```python
from build123d import *

# Parameters (mm, degrees)
SKETCH1_W               = 450
SKETCH1_H               = 280
BOSS_EXTRUDE1_DEPTH     = 95
FILLET1_R               = 10
FILLET2_R               = 5
CUT_EXTRUDE1_DEPTH      = 89
BOSS_EXTRUDE2_REACH     = 283.514
MIRROR2_COPY_1_REACH    = 283.514
FILLET4_R               = 1
SKETCH7_R               = 4
CUT_EXTRUDE2_DEPTH      = 40
MIRROR4_COPY_1_SKETCH_R = 4
MIRROR4_COPY_1_DEPTH    = 40
SKETCH8_R               = 2.25
SKETCH8_W               = 47
SKETCH8_H               = 26.9
CUT_EXTRUDE3_DEPTH      = 10
SKETCH10_R              = 2.53
SLOTS_FOR_LEDS_DEPTH    = 10
SKETCH11_R              = 12
SKETCH11_R_2            = 1.6
CUT_EXTRUDE4_DEPTH      = 10
SKETCH12_R              = 12
SKETCH12_R_2            = 1.6
CUT_EXTRUDE5_DEPTH      = 10


with BuildPart() as part:
    # Sketch1 → Boss-Extrude1 (new body)
    with BuildSketch(Plane(origin=(0, 0, 0), x_dir=(1, 0, 0), z_dir=(0, 1, 0))):
        Rectangle(SKETCH1_W, SKETCH1_H)
    extrude(amount=BOSS_EXTRUDE1_DEPTH)

    # Fillet1
    fillet1_edges = [part.edges().sort_by_distance(p)[0] for p in [
        (225, 47.5, 140),
        (-225, 47.5, 140),
        (-225, 47.5, -140),
        (225, 47.5, -140),
    ]]
    fillet(fillet1_edges, radius=FILLET1_R)

    # Fillet2
    fillet2_edges = [part.edges().sort_by_distance(p)[0] for p in [
        (-225, 0, 0),
        (225, 0, 0),
        (0, 0, 140),
        (0, 0, -140),
        (-222.071067812, 0, 137.071067812),
        (222.071067812, 0, 137.071067812),
        (222.071067812, 0, -137.071067812),
        (-222.071067812, 0, -137.071067812),
    ]]
    fillet(fillet2_edges, radius=FILLET2_R)

    # Sketch3 → Cut-Extrude1 (cut)
    with BuildSketch(Plane(origin=(0, 95, 0), x_dir=(1, 0, 0), z_dir=(0, 1, 0))):
        with BuildLine():
            Line((220, -130), (220, 130))
            ThreePointArc((220, 130), (218.535533906, 133.535533906), (215, 135))
            Line((215, 135), (-215, 135))
            ThreePointArc((-215, 135), (-218.535533906, 133.535533906), (-220, 130))
            Line((-220, 130), (-220, -130))
            ThreePointArc((-220, -130), (-218.535533906, -133.535533906), (-215, -135))
            Line((-215, -135), (215, -135))
            ThreePointArc((215, -135), (218.535533906, -133.535533906), (220, -130))
        make_face()
    extrude(amount=-CUT_EXTRUDE1_DEPTH, mode=Mode.SUBTRACT)

    # Sketch5 → Boss-Extrude2 (add, up to next)
    with BuildSketch(Plane(origin=(0, 95, 0), x_dir=(1, 0, 0), z_dir=(0, 1, 0)), mode=Mode.PRIVATE) as boss_extrude2_sk1:
        with BuildLine():
            Line((-205, 135), (-215, 135))
            ThreePointArc((-215, 135), (-218.535533906, 133.535533906), (-220, 130))
            Line((-220, 130), (-220, 120))
            ThreePointArc((-220, 120), (-209.393398282, 124.393398282), (-205, 135))
        make_face()
    boss_extrude2_tool1 = extrude(boss_extrude2_sk1.sketch, amount=-BOSS_EXTRUDE2_REACH, mode=Mode.PRIVATE) - part.part
    boss_extrude2 = boss_extrude2_tool1.solids().sort_by_distance((-213.469442, 95, -128.469442))[0]
    add(boss_extrude2)

    # Mirror1: Boss-Extrude2 across plane
    add(boss_extrude2.mirror(Plane.XY))

    # Mirror2: Boss-Extrude2 across plane
    add(boss_extrude2.mirror(Plane(origin=(0, 0, 0), x_dir=(0, 0, 1), z_dir=(1, 0, 0))))

    # Mirror2 copy 1 sketch → Mirror2 copy 1 (add, up to next)
    with BuildSketch(Plane(origin=(0, 95, 0), x_dir=(-1, 0, 0), z_dir=(0, 1, 0)), mode=Mode.PRIVATE) as mirror2_copy_1_sk1:
        with BuildLine():
            Line((-205, 135), (-215, 135))
            ThreePointArc((-215, 135), (-218.535533906, 133.535533906), (-220, 130))
            Line((-220, 130), (-220, 120))
            ThreePointArc((-220, 120), (-209.393398282, 124.393398282), (-205, 135))
        make_face()
    mirror2_copy_1_tool1 = extrude(mirror2_copy_1_sk1.sketch, amount=-MIRROR2_COPY_1_REACH, mode=Mode.PRIVATE) - part.part
    add(mirror2_copy_1_tool1.solids().sort_by_distance((213.469442, 95, 128.469442))[0])

    # Fillet4
    fillet4_edges = [part.edges().sort_by_distance(p)[0] for p in [
        (-220, 6, 0),
        (-209.393398282, 6, 124.393398282),
        (0, 6, 135),
        (209.393398282, 6, 124.393398282),
        (220, 6, 0),
        (209.393398282, 6, -124.393398282),
        (0, 6, -135),
        (-209.393398282, 6, -124.393398282),
    ]]
    fillet(fillet4_edges, radius=FILLET4_R)

    # Sketch7 → Cut-Extrude2 (cut)
    with BuildSketch(Plane(origin=(0, 95, 0), x_dir=(1, 0, 0), z_dir=(0, 1, 0))):
        with Locations(Location((-215, 130, 0), (0, 0, 270))):
            Circle(SKETCH7_R)
    cut_extrude2 = extrude(amount=-CUT_EXTRUDE2_DEPTH, mode=Mode.SUBTRACT)

    # Mirror3: Cut-Extrude2 across plane
    add(cut_extrude2.mirror(Plane.XY), mode=Mode.SUBTRACT)

    # Mirror4: Cut-Extrude2 across plane
    add(cut_extrude2.mirror(Plane(origin=(0, 0, 0), x_dir=(0, 0, 1), z_dir=(1, 0, 0))), mode=Mode.SUBTRACT)

    # Mirror4 copy 1 sketch → Mirror4 copy 1 (cut)
    with BuildSketch(Plane(origin=(0, 95, 0), x_dir=(-1, 0, 0), z_dir=(0, 1, 0))):
        with Locations(Location((-215, 130, 0), (0, 0, 270))):
            Circle(MIRROR4_COPY_1_SKETCH_R)
    extrude(amount=-MIRROR4_COPY_1_DEPTH, mode=Mode.SUBTRACT)

    # Sketch8 → Cut-Extrude3 (cut)
    with BuildSketch(Plane.XY.offset(140)):
        with Locations((-183, 35)):
            Circle(SKETCH8_R)
        with Locations((-127, 35)):
            Circle(SKETCH8_R)
        with Locations((-155, 35)):
            Rectangle(SKETCH8_W, SKETCH8_H)
    extrude(amount=-CUT_EXTRUDE3_DEPTH, mode=Mode.SUBTRACT)

    # Sketch10 → Slots for LEDs (cut)
    with BuildSketch(Plane(origin=(0, 0, -140), x_dir=(-1, 0, 0), z_dir=(0, 0, -1))):
        with Locations((-17, 75)):
            Circle(SKETCH10_R)
        with Locations((-2, 75)):
            Circle(SKETCH10_R)
        with Locations((13, 75)):
            Circle(SKETCH10_R)
        with Locations((28, 75)):
            Circle(SKETCH10_R)
        with Locations((43, 75)):
            Circle(SKETCH10_R)
        with Locations((58, 75)):
            Circle(SKETCH10_R)
    extrude(amount=-SLOTS_FOR_LEDS_DEPTH, mode=Mode.SUBTRACT)

    # Sketch11 → Cut-Extrude4 (cut)
    with BuildSketch(Plane.XY.offset(140)):
        with Locations((63.955734546, 69.39400536)):
            Circle(SKETCH11_R)
        with Locations((73.455734546, 41.39400536)):
            Circle(SKETCH11_R_2)
        with Locations((54.455734546, 17.39400536)):
            Circle(SKETCH11_R_2)
        with Locations((113.955734546, 69.39400536)):
            Circle(SKETCH11_R)
        with Locations((113.955734546, 29.39400536)):
            Circle(SKETCH11_R)
        with Locations((63.955734546, 29.39400536)):
            Circle(SKETCH11_R)
        with Locations((73.455734546, 81.39400536)):
            Circle(SKETCH11_R_2)
        with Locations((54.455734546, 57.39400536)):
            Circle(SKETCH11_R_2)
        with Locations((123.455734546, 41.39400536)):
            Circle(SKETCH11_R_2)
        with Locations((104.455734546, 17.39400536)):
            Circle(SKETCH11_R_2)
        with Locations((123.455734546, 81.39400536)):
            Circle(SKETCH11_R_2)
        with Locations((104.455734546, 57.39400536)):
            Circle(SKETCH11_R_2)
    extrude(amount=-CUT_EXTRUDE4_DEPTH, mode=Mode.SUBTRACT)

    # Sketch12 → Cut-Extrude5 (cut)
    with BuildSketch(Plane(origin=(0, 0, -140), x_dir=(-1, 0, 0), z_dir=(0, 0, -1))):
        with Locations((-67.078371633, 71.762757401)):
            Circle(SKETCH12_R)
        with Locations((-80.078371633, 84.762757401)):
            Circle(SKETCH12_R_2)
        with Locations((-54.078371633, 58.762757401)):
            Circle(SKETCH12_R_2)
        with Locations((-80.078371633, 44.762757401)):
            Circle(SKETCH12_R_2)
        with Locations((-67.078371633, 31.762757401)):
            Circle(SKETCH12_R)
        with Locations((-54.078371633, 18.762757401)):
            Circle(SKETCH12_R_2)
        with Locations((-54.078371633, 84.762757401)):
            Circle(SKETCH12_R_2)
        with Locations((-80.078371633, 58.762757401)):
            Circle(SKETCH12_R_2)
        with Locations((-54.078371633, 44.762757401)):
            Circle(SKETCH12_R_2)
        with Locations((-80.078371633, 18.762757401)):
            Circle(SKETCH12_R_2)
    extrude(amount=-CUT_EXTRUDE5_DEPTH, mode=Mode.SUBTRACT)


solid = part.part
```
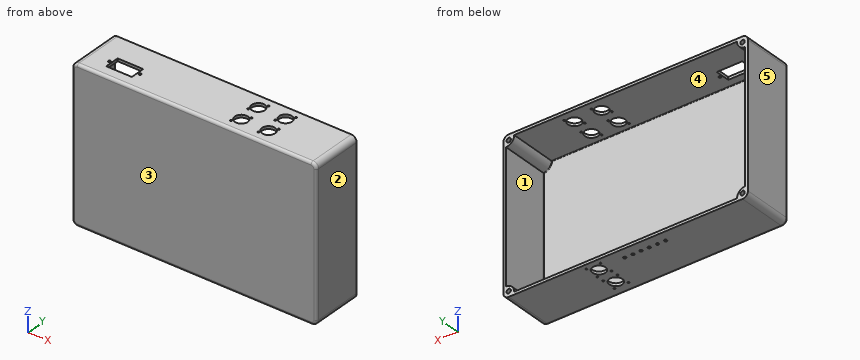
For this review, take the finished solid that the model builds, in its own axes (mm). Face numbers are marked on the shaded views. A direction names the side the tool comes from. Round coordinates to 2 decimals unless told otherwise and drop trailing zeros. Write each loop counter-clockwise with the first axis right and the second up, starting at its lowest first coordinate (ties: lowest second). Pieces come first, ordered by that corner, then holes. Notation, with made-up numbers: (32, 36.5) -> (79, 36.5) arc R32 cw to (79, 74.5) -> close; hole circle Ø6 at (67, -30.75). An arc over 180 degrees is marked (long way). One line per question, with ' | ' between items. Start each with the question number.
(1) Tool access review of the marked faces 1 and 2: name each direction out of +Z, -Z, +X, -X, +Y, -Y from which nothing blocks a thin tool from reaching the whole face with its end or side.
(2) Mouldability with a two-part tool opening along X and no side actions: class the marked faces 3, 4 and 5 as released by +X, released by -X, zero draft, split by the parting line, or undercut.
(3) Add section B-B, the plane z = 37. Write out the cut boundary in (x, y).
(4) Insertion check: P1, Ø4.5, axis at x = 17, y = 75, coming from the -Z side; P2, Ø5, axis at x = 215, z = -130, coming from the +Y side; P3, Ø2.5, axis at x = 54.46, y = 17.39, coming from the +Z side. Each pin has a flat end and moves straight along its axis. Give the tip position at first contact, or say it passes through.
(5) For line 1 along Z through (x, y) = (42.5, 67); line 2 along X through (y, z) = (47, -28.5); line 3 along Z through (x, y) = (215, 70), list the stretches that pass through material, from the lowest coordinate up. Write a range as from..to.
(6) Add section A-A, the plane x = 44. Write out the cut boundary in (y, z), plus the area to 3 significant figures.
Answer list:
1) face 1: +Y | face 2: +Z, -Z, +X, +Y, -Y
2) face 3: zero draft | face 4: undercut | face 5: released by -X
3) outline: (-225, 5) arc R5 ccw to (-220, 0) -> (220, 0) arc R5 ccw to (225, 5) -> (225, 95) -> (220, 95) -> (220, 7) arc R1 cw to (219, 6) -> (-219, 6) arc R1 cw to (-220, 7) -> (-220, 95) -> (-225, 95) -> close
4) P1: z = 135 | P2: y = 55 | P3: z = -135
5) line 1: -140..-135, 135..140 | line 2: -225..-220, 220..225 | line 3: -140..-134, -126..-120.86, 120.86..126, 134..140
6) outline: (0, -135) arc R5 ccw to (5, -140) -> (95, -140) -> (95, -135) -> (7, -135) arc R1 cw to (6, -134) -> (6, 134) arc R1 cw to (7, 135) -> (95, 135) -> (95, 140) -> (5, 140) arc R5 ccw to (0, 135) -> close | area: 2,560 mm²
